For this review, use the dimensioned drawing (mm, ordinates from the lowest corner) and the shaded views. Coordinates: 2 decimals unless noted, no trailing zeros. Loops run counter-clockwise (first coordinate to the right, second up) from the corner with the lowest first, then second, coordinate; pieces in that order, holes last. Notation, with made-up numbers: (47.25, 25) - (97.25, 25) arc R18 cw to (97.25, 48) - close; hole circle Ø11 at (-9, 53.5). An arc over 180 degrees is marked (long way). Answer in a Markdown table with one row per item. Add a question column.
(1) We need section C-C, the plane z = 1.3. Write out the cut boundary in (x, y), plus the area to 3 significant figures.
(2) We need section A-A, the plane x = 4.5. Write out the cut boundary in (y, z), plus the area to 3 significant figures.
(3) We need section D-D, the plane z = 0.3. Write out the cut boundary in (x, y), plus the area to 3 significant figures.
(4) The part is to be moulded in two halves that separate along Y. For the marked faces 1, 2 and 3, say which applies: released by +Y, released by -Y, zero draft, split by the parting line, or undercut.
(5) To check wall thickness, follow L1, parallel to Y at x = 4.5, z = 1.7; L2, parallel to Y at x = 5, z = 3.6; L3, parallel to X at y = 6.25, z = 4.15. State the ranges of each line that lie inside material, in increasing order. Write a range as [from, to].
(6) Clearance check with flat-ended pins moving along their axes: pin 1 (4 mm diameter, centred on x = 5.5, y = 2, fed in from +Z); pin 2 (2 mm diameter, centred on y = 7.5, z = 2.5, fed in from -X); pin 3 (2 mm diameter, centred on x = 4.5, y = 4.5, fed in from +Z); pin 4 (2 mm diameter, centred on y = 6.5, z = 2, fed in from +X). State where each tip first meets the part, or that it passes through.
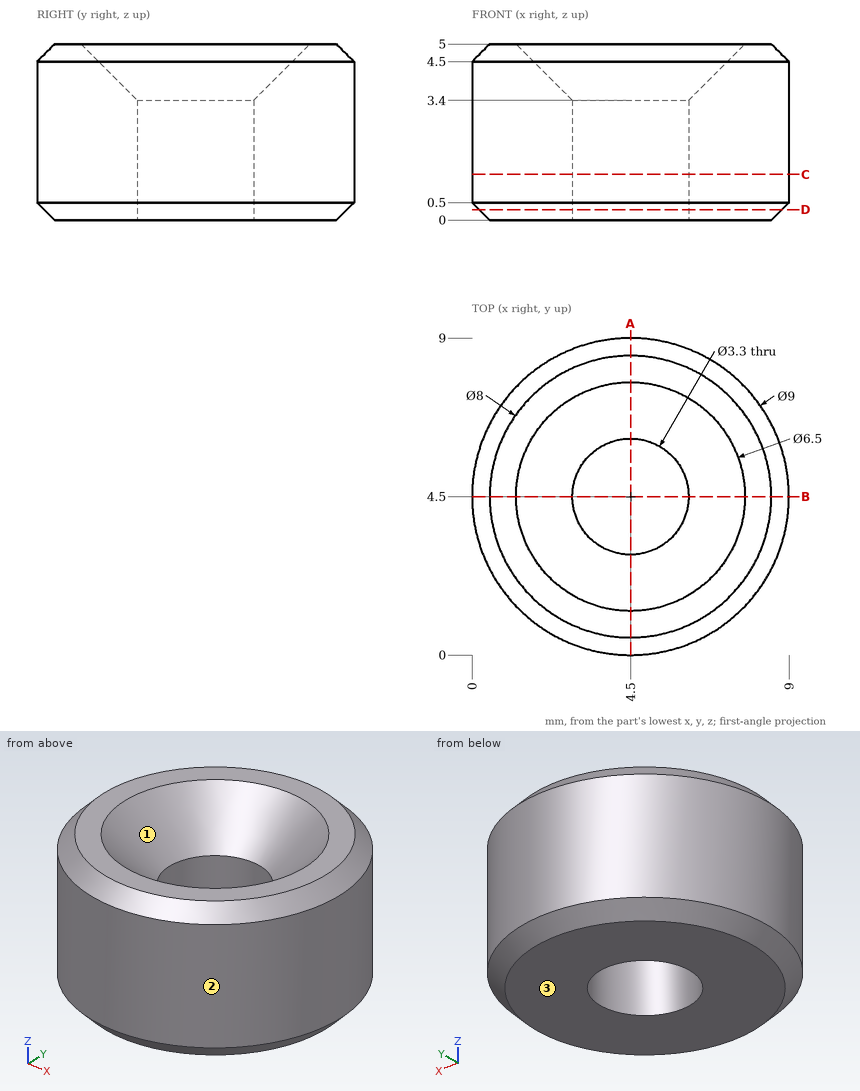
Responses:
| question | item | result |
|---|---|---|
| 1 | outline | circle Ø9 at (4.5, 4.5); hole circle Ø3.3 at (4.5, 4.5) |
| 1 | area | 55.1 mm2 |
| 2 | outline | (0, 0.5) - (0.5, 0) - (2.85, 0) - (2.85, 3.4) - (1.25, 5) - (0.5, 5) - (0, 4.5) - close; (6.15, 0) - (8.5, 0) - (9, 0.5) - (9, 4.5) - (8.5, 5) - (7.75, 5) - (6.15, 3.4) - close |
| 2 | area | 25.4 mm2 |
| 3 | outline | circle Ø8.6 at (4.5, 4.5); hole circle Ø3.3 at (4.5, 4.5) |
| 3 | area | 49.5 mm2 |
| 4 | face 1 | undercut |
| 4 | face 2 | split by the parting line |
| 4 | face 3 | zero draft |
| 5 | L1 | y = [0, 2.85], [6.15, 9] |
| 5 | L2 | y = [0.03, 2.72], [6.28, 8.97] |
| 5 | L3 | x = [0.35, 2.86], [6.14, 8.65] |
| 6 | pin 1 | stops at z = 5 |
| 6 | pin 2 | stops at x = 0.47 |
| 6 | pin 3 | passes through |
| 6 | pin 4 | stops at x = 8.89 |
